The model under review builds one solid part; all positions refer to its coordinate system, in mm. A direction names the side the tool comes from. Round coordinates to 2 decimals unless told otherwise and drop trailing zeros. Write each loop counter-clockwise with the first axis right and the second up, starting at its lowest first coordinate (ties: lowest second). Pieces come first, ordered by that corner, then holes. Notation, with made-up numbers: (5.25, 19.5) -> (9.25, 19.5) arc R21 cw to (9.25, 38.5) -> close; hole circle Ø4 at (-27.5, 68.5). An arc over 180 degrees is marked (long way). Answer as a JSON object with one key per item and string values. Group by question number.
1) We need section A-A, the plane x = 15. Write out the cut boundary in (y, z).
2) We need section B-B, the plane y = -12.5. Write out the cut boundary in (x, z), then the cut area to 3 significant figures.
3) We need section C-C, the plane x = -24.5. Write out the cut boundary in (y, z), then the cut area to 3 significant figures.
4) Insertion check: pin 1 Ø8 at (x, y) = (15, 12.5) entering from -Z; pin 2 Ø3 at (x, y) = (-14, 12.5) entering from +Z; pin 3 Ø3 at (x, z) = (22, 8.5) entering from +Y; pin 4 Ø2.5 at (x, y) = (24, 1) entering from -Z. Each pin has a flat end and moves straight along its axis. Give the tip position at first contact, or say it passes through.
5) We need section D-D, the plane y = -7. Write out the cut boundary in (x, z), then the cut area to 3 significant figures.
6) To check wall thickness, follow probe 1 along Y at (x, z) = (-15, 2.8); probe 2 along Y at (x, z) = (15, 10.15); probe 3 along Y at (x, z) = (7, 2.25). State the ranges of each line that lie inside material, in increasing order. Write a range as [from, to].
7) Mouldability with a two-part tool opening along X and no side actions: class faces 4 (the flat face through (26.3, 11.2, 5.4)), 5 (the flat face through (0, 0, 12)), 6 (the cylindrical face through (-18, 12.6, 9)) as pulls with the +X half, pulls with the -X half, needs draft (parallel to the pull), parting line crosses it, or undercut.
8) Machinability: for faces 1 (the cylindrical face through (0.1, 16.1, 6.5)), 2 (the flat face through (-14, -14, 6)), 3 (the cylindrical face through (19.3, -2.4, 2.5)), which of the approach directions +Z, -Z, +X, -X, +Y, -Y give a long, thin tool a straight path to every point of the face, cutting with its end or side? Answer none if there is none.
from build123d import *

# Parameters (mm, degrees)
SKETCH_R          = 1.6
PAD_DEPTH         = 12
SKETCH001_R       = 6.5
POCKET_DEPTH      = 17.501
POCKET_DEPTH_BACK = -17.501
SKETCH002_R       = 9.6
POCKET001_DEPTH   = 14.75
SKETCH003_R       = 3
POCKET002_DEPTH   = 6
SKETCH004_R       = 4
POCKET003_DEPTH   = 5
CHAMFER_SIZE      = 1


with BuildPart() as part:
    # Sketch → Pad (new body)
    with BuildSketch(Plane.XY):
        Polygon((-32.5, 5), (-32.5, -5), (-20, -17.5), (20, -17.5), (32.5, -5), (32.5, 5), (20, 17.5), (-20, 17.5), align=None)
        with Locations((-15, 12.5)):
            Circle(SKETCH_R, mode=Mode.SUBTRACT)
        with Locations((15, 12.5)):
            Circle(SKETCH_R, mode=Mode.SUBTRACT)
        with Locations((-15, -12.5)):
            Circle(SKETCH_R, mode=Mode.SUBTRACT)
        with Locations((15, -12.5)):
            Circle(SKETCH_R, mode=Mode.SUBTRACT)
    extrude(amount=PAD_DEPTH)

    # Sketch001 → Pocket (cut, two sides)
    with BuildSketch(Plane.XZ) as pocket_sk:
        Circle(SKETCH001_R)
    extrude(amount=-POCKET_DEPTH, mode=Mode.SUBTRACT)
    extrude(pocket_sk.sketch, amount=-POCKET_DEPTH_BACK, mode=Mode.SUBTRACT)

    # Sketch002 → Pocket001 (cut, symmetric)
    with BuildSketch(Plane.XZ):
        Circle(SKETCH002_R)
    extrude(amount=POCKET001_DEPTH, both=True, mode=Mode.SUBTRACT)

    # Sketch003 (on Face5 of Pocket001) → Pocket002 (cut)
    with BuildSketch(Plane.XY.offset(12)):
        with Locations((-15, 12.5)):
            Circle(SKETCH003_R)
        with Locations((15, 12.5)):
            Circle(SKETCH003_R)
        with Locations((-15, -12.5)):
            Circle(SKETCH003_R)
        with Locations((15, -12.5)):
            Circle(SKETCH003_R)
    extrude(amount=-POCKET002_DEPTH, mode=Mode.SUBTRACT)

    # Sketch004 → Pocket003 (cut)
    with BuildSketch(Plane.XY):
        with Locations((-22.5, 0)):
            Circle(SKETCH004_R)
        with Locations((22.5, 0)):
            Circle(SKETCH004_R)
    extrude(amount=POCKET003_DEPTH, mode=Mode.SUBTRACT)

    # Chamfer
    chamfer_edges = [part.edges().sort_by_distance(p)[0] for p in [
        (0, 17.5, 12),
        (-26.25, 11.25, 12),
        (-32.5, 0, 12),
        (-26.25, -11.25, 12),
        (0, -17.5, 12),
        (26.25, -11.25, 12),
        (32.5, 0, 12),
        (26.25, 11.25, 12),
    ]]
    chamfer(chamfer_edges, length=CHAMFER_SIZE)


solid = part.part
Here are the results:
{
 "1": {"outline": "(-17.5, 0) -> (-14.1, 0) -> (-14.1, 6) -> (-15.5, 6) -> (-15.5, 12) -> (-16.5, 12) -> (-17.5, 11) -> close; (-10.9, 0) -> (10.9, 0) -> (10.9, 6) -> (9.5, 6) -> (9.5, 12) -> (-9.5, 12) -> (-9.5, 6) -> (-10.9, 6) -> close; (14.1, 0) -> (17.5, 0) -> (17.5, 11) -> (16.5, 12) -> (15.5, 12) -> (15.5, 6) -> (14.1, 6) -> close"},
 "2": {"outline": "(-25, 0) -> (-16.6, 0) -> (-16.6, 6) -> (-18, 6) -> (-18, 12) -> (-23.59, 12) -> (-25, 11) -> close; (-13.4, 0) -> (-9.6, 0) arc R9.6 cw to (9.6, 0) -> (13.4, 0) -> (13.4, 6) -> (12, 6) -> (12, 12) -> (-12, 12) -> (-12, 6) -> (-13.4, 6) -> close; (16.6, 0) -> (25, 0) -> (25, 11) -> (23.59, 12) -> (18, 12) -> (18, 6) -> (16.6, 6) -> close", "area": "343 mm^2"},
 "3": {"outline": "(-13, 0) -> (-3.46, 0) -> (-3.46, 5) -> (3.46, 5) -> (3.46, 0) -> (13, 0) -> (13, 11) -> (11.59, 12) -> (-11.59, 12) -> (-13, 11) -> close", "area": "276 mm^2"},
 "4": {"pin 1": "stops at z = 0", "pin 2": "stops at z = 6", "pin 3": "stops at y = 17", "pin 4": "stops at z = 5"},
 "5": {"outline": "(-30.5, 0) -> (-9.6, 0) arc R9.6 cw to (9.6, 0) -> (30.5, 0) -> (30.5, 11) -> (29.09, 12) -> (-29.09, 12) -> (-30.5, 11) -> close", "area": "586 mm^2"},
 "6": {"probe 1": "y = [-17.5, -14.1], [-10.9, 10.9], [14.1, 17.5]", "probe 2": "y = [-17.5, -15.5], [-9.5, 9.5], [15.5, 17.5]", "probe 3": "y = [-17.5, -14.75], [14.75, 17.5]"},
 "7": {"face 4": "pulls with the +X half", "face 5": "needs draft", "face 6": "undercut"},
 "8": {"face 1": "-Z, +Y, -Y", "face 2": "+Z", "face 3": "-Z"}
}
